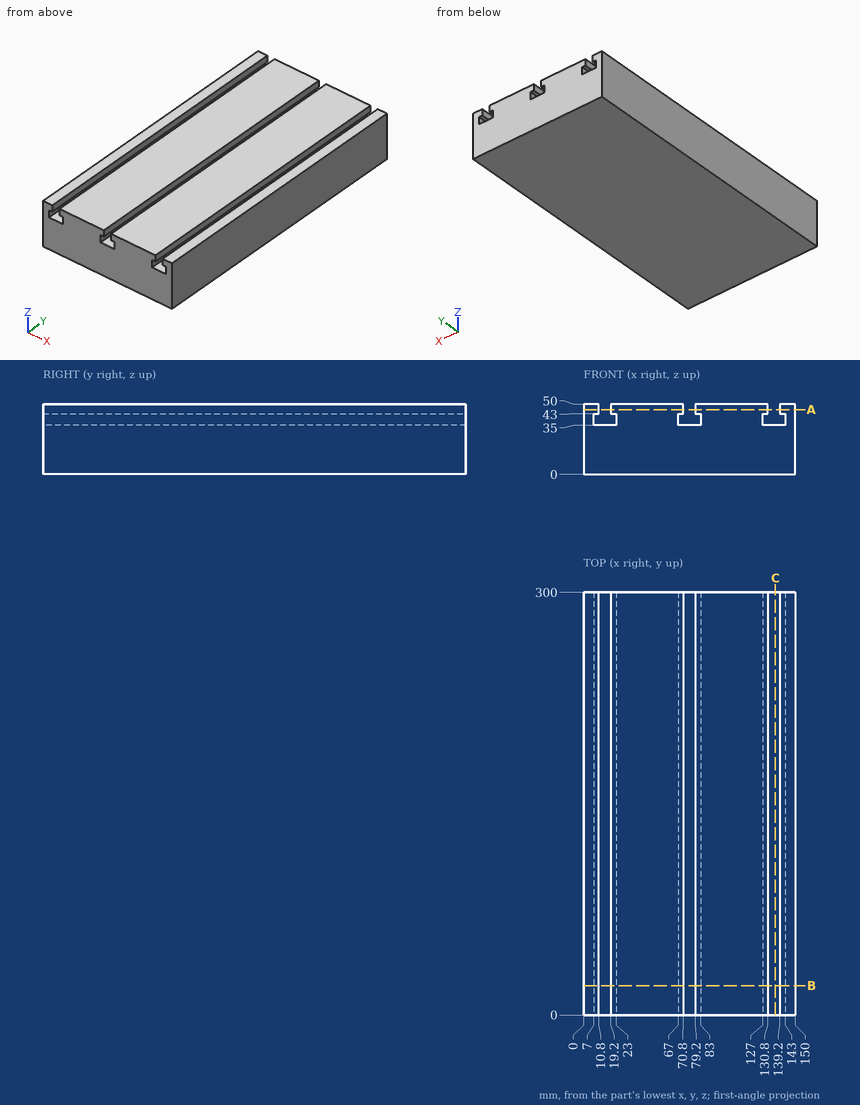
Job drawing, mm, ordinate dimensions from the low corner. One solid piece. Coordinates: 2 decimals unless noted, no trailing zeros. Write each loop counter-clockwise with the first axis right and the second up, starting at its lowest first coordinate (ties: lowest second). Pieces come first, ordered by that corner, then holes.
Item 1: Probe line 1 (X direction, y = 95, z = 41); line 2 (Z direction, x = 70, y = 77); line 3 (Z direction, x = 77.5, y = 222.5). List the from-to ranges inside material, lowest first.
Item 2: Pin check, flat tip, straight feed: pin 1 (1.9 mm diameter, centred on x = 69.5, y = 201.5, fed in from -Z). Stop position of the tip, or through.
Item 3: Slice it at C-C (x = 136). Write the cut outline in (y, z), and give its area (3 significant figures).
Item 4: Slice it at B-B (y = 21). Write the cut outline in (x, z).
Item 5: Slice it at A-A (z = 46). Write the cut outline in (x, y).
Results found:
1. line 1: x = 0 to 7, 23 to 67, 83 to 127, 143 to 150
1. line 2: z = 0 to 35, 43 to 50
1. line 3: z = 0 to 35
2. pin 1: stops at z = 0
3. outline: (0, 0) - (300, 0) - (300, 35) - (0, 35) - close
3. area: 10,500 mm2
4. outline: (0, 0) - (150, 0) - (150, 50) - (139.2, 50) - (139.2, 43) - (143, 43) - (143, 35) - (127, 35) - (127, 43) - (130.8, 43) - (130.8, 50) - (79.2, 50) - (79.2, 43) - (83, 43) - (83, 35) - (67, 35) - (67, 43) - (70.8, 43) - (70.8, 50) - (19.2, 50) - (19.2, 43) - (23, 43) - (23, 35) - (7, 35) - (7, 43) - (10.8, 43) - (10.8, 50) - (0, 50) - close
5. outline: (0, 0) - (10.8, 0) - (10.8, 300) - (0, 300) - close; (19.2, 0) - (70.8, 0) - (70.8, 300) - (19.2, 300) - close; (79.2, 0) - (130.8, 0) - (130.8, 300) - (79.2, 300) - close; (139.2, 0) - (150, 0) - (150, 300) - (139.2, 300) - close
